Design review of the part built by this model. Coordinates are the model's own, in mm. Coordinates: 2 decimals unless noted, no trailing zeros. Loops run counter-clockwise (first coordinate to the right, second up) from the corner with the lowest first, then second, coordinate; pieces in that order, holes last.
Q1. Wall thickness on probe 1 along X at (y, z) = (2.1, -218.5); probe 2 along X at (y, z) = (0.2, -343); probe 3 along Z at (x, y) = (-53.5, 1.5): over which ranges is each line inside the solid? List them lowest first.
Q2. For P1, Ø0.9, axis at x = 66.5, y = 1, coming from the -Z side; P2, Ø1, axis at x = -54, y = 2.5, coming from the -Z side; P3, Ø0.9, axis at x = 23.5, y = 1, coming from the +Z side, all flat-tipped, find the tip position at first contact; note any pin that passes through.
Q3. Add section C-C on x = 69.5. Give the boundary of the cut face in (y, z).
Q4. Add section A-A on y = 0.7. Give the number of separate pieces and of enclosed holes in the cut face, and give its area (3 significant figures).
Q5. Add section B-B on z = -203.5. Give the boundary of the cut face in (x, y).
```python
from build123d import *

# Parameters (mm, degrees)
SKETCH1_W           = 3
SKETCH1_H           = 30
BOSS_EXTRUDE1_DEPTH = 3


with BuildPart() as part:
    # Sketch1 → Boss-Extrude1 (new body)
    with BuildSketch(Plane(origin=(0, 0, 0), x_dir=(1, 0, 0), z_dir=(0, 1, 0))):
        Polygon((31, 456), (42, 456), (42, 100), (82, 100), (131, 60), (131, 0), (31, 0), (31, 3), (11, 3), (11, 0), (-89, 0), (-89, 60), (-40, 100), (0, 100), (0, 456), (11, 456), (11, 453), (31, 453), align=None)
        with Locations((37.5, 68)):
            Rectangle(SKETCH1_W, SKETCH1_H, mode=Mode.SUBTRACT)
        with Locations((37.5, 228)):
            Rectangle(SKETCH1_W, SKETCH1_H, mode=Mode.SUBTRACT)
        with Locations((37.5, 388)):
            Rectangle(SKETCH1_W, SKETCH1_H, mode=Mode.SUBTRACT)
        with Locations((4.5, 68)):
            Rectangle(SKETCH1_W, SKETCH1_H, mode=Mode.SUBTRACT)
        with Locations((4.5, 228)):
            Rectangle(SKETCH1_W, SKETCH1_H, mode=Mode.SUBTRACT)
        with Locations((4.5, 388)):
            Rectangle(SKETCH1_W, SKETCH1_H, mode=Mode.SUBTRACT)
    extrude(amount=BOSS_EXTRUDE1_DEPTH)


solid = part.part
```
Entries:
1. probe 1: x = 0 to 3, 6 to 36, 39 to 42
1. probe 2: x = 0 to 42
1. probe 3: z = -88.98 to 0
2. P1: stops at z = -100
2. P2: stops at z = -88.98
2. P3: stops at z = -3
3. outline: (0, -100) - (3, -100) - (3, 0) - (0, 0) - close
4. separate pieces: 1
4. enclosed holes: 6
4. area: 34,300 mm2
5. outline: (0, 0) - (42, 0) - (42, 3) - (0, 3) - close
